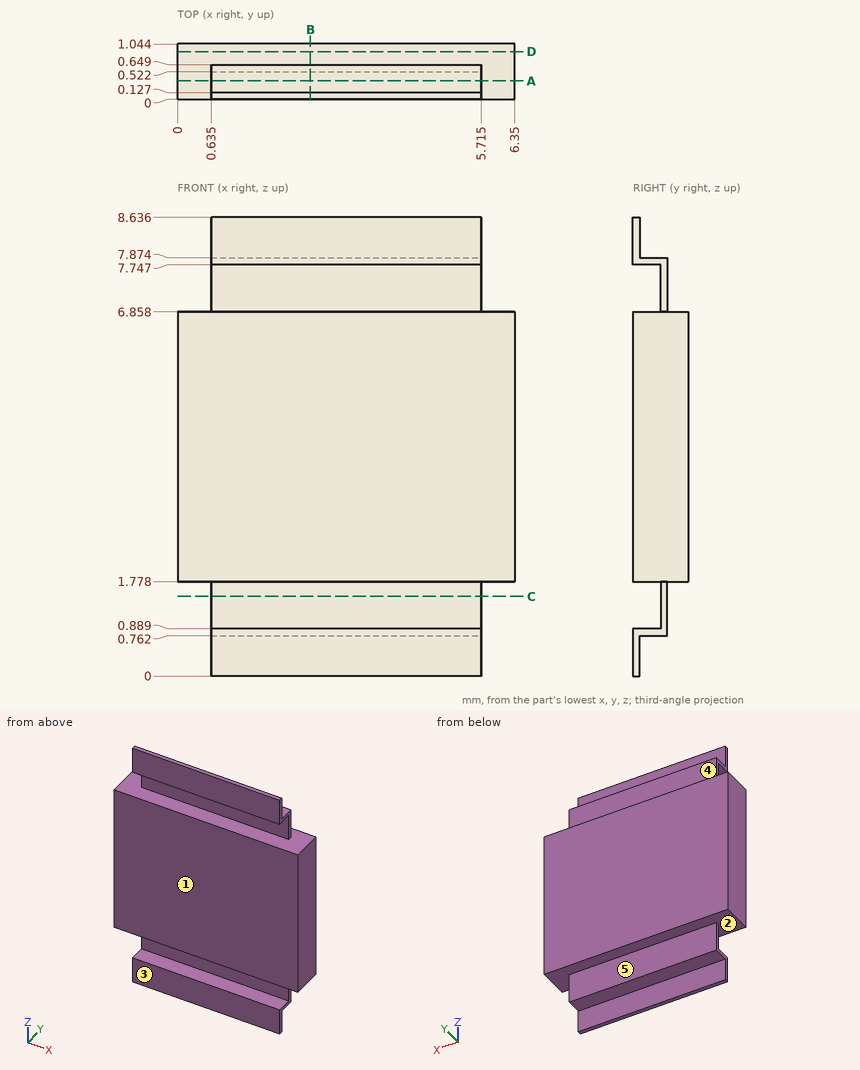
Can you work these out from the drawing? Everything is in mm from the part's minimum corner. A direction names the side the tool comes from. Coordinates: 2 decimals unless noted, no trailing zeros. Loops run counter-clockwise (first coordinate to the right, second up) from the corner with the lowest first, then second, coordinate; pieces in that order, holes last. Notation, with made-up numbers: (-13.5, 10.5) - (7.5, 10.5) arc R14 cw to (7.5, 17.5) - close; hole circle Ø9 at (-25, 70.5). An arc over 180 degrees is marked (long way). Put each result on its own line as item: value. Start each with the question number.
Item 1: For pin 1 (0.6 mm diameter, centred on x = 2.5, y = 0, fed in from -Z); pin 2 (0.8 mm diameter, centred on x = 3, z = 8.5, fed in from +Y); pin 3 (0.5 mm diameter, centred on x = 4.5, y = 0.5, fed in from -Z), each with a flat end and sliding along its axis, tell me the tip position at first contact or that it passes through.
Item 2: If we mould it in two halves opening along Z, with no side actions, what happens to the marked faces 1 and 2? For each: +Z half, -Z half, draft (parallel to the pull), parting line (faces both ways), or undercut.
Item 3: If I drill on line 1 along Z through (x, y) = (4.5, 0.85), over which ranges is the centre line in solid material (lowest first)?
Item 4: Suppose I cut it at A-A (y = 0.35). Please give me the cut outline in (x, z) (3 decimals), and give its area (3 significant figures).
Item 5: Which directions (+Z, -Z, +X, -X, +Y, -Y) give clear straight access to the entire face, cutting with the end or side of a thin tool? Please do the marked faces 3, 4 and 5.
Item 6: Suppose I cut it at C-C (z = 1.5). Please give me the cut outline in (x, y) (3 decimals), and give its area (3 significant figures).
Item 7: Suppose I cut it at D-D (y = 0.9). Please give me the cut outline in (x, z), and give its area (3 significant figures).
Item 8: Suppose I cut it at B-B (x = 2.5). Please give me the cut outline in (y, z), and give its area (3 significant figures).
Here are the results:
1. pin 1: z = 0
1. pin 2: y = 0.13
1. pin 3: z = 0.76
2. face 1: draft
2. face 2: undercut
3. line 1: 1.78 to 6.86
4. outline: (0, 1.778) - (6.35, 1.778) - (6.35, 6.858) - (0, 6.858) - close; (0.635, 0.762) - (5.715, 0.762) - (5.715, 0.889) - (0.635, 0.889) - close; (0.635, 7.747) - (5.715, 7.747) - (5.715, 7.874) - (0.635, 7.874) - close
4. area: 33.5 mm²
5. face 3: +Z, -Z, +X, -X, -Y
5. face 4: +Z, +X, -X, +Y
5. face 5: -Z, +X, -X, +Y
6. outline: (0.635, 0.522) - (5.715, 0.522) - (5.715, 0.649) - (0.635, 0.649) - close
6. area: 0.645 mm²
7. outline: (0, 1.78) - (6.35, 1.78) - (6.35, 6.86) - (0, 6.86) - close
7. area: 32.3 mm²
8. outline: (0, 0) - (0.13, 0) - (0.13, 0.76) - (0.65, 0.76) - (0.65, 1.78) - (1.04, 1.78) - (1.04, 6.86) - (0.65, 6.86) - (0.65, 7.87) - (0.13, 7.87) - (0.13, 8.64) - (0, 8.64) - (0, 7.75) - (0.52, 7.75) - (0.52, 6.86) - (0, 6.86) - (0, 1.78) - (0.52, 1.78) - (0.52, 0.89) - (0, 0.89) - close
8. area: 5.89 mm²
